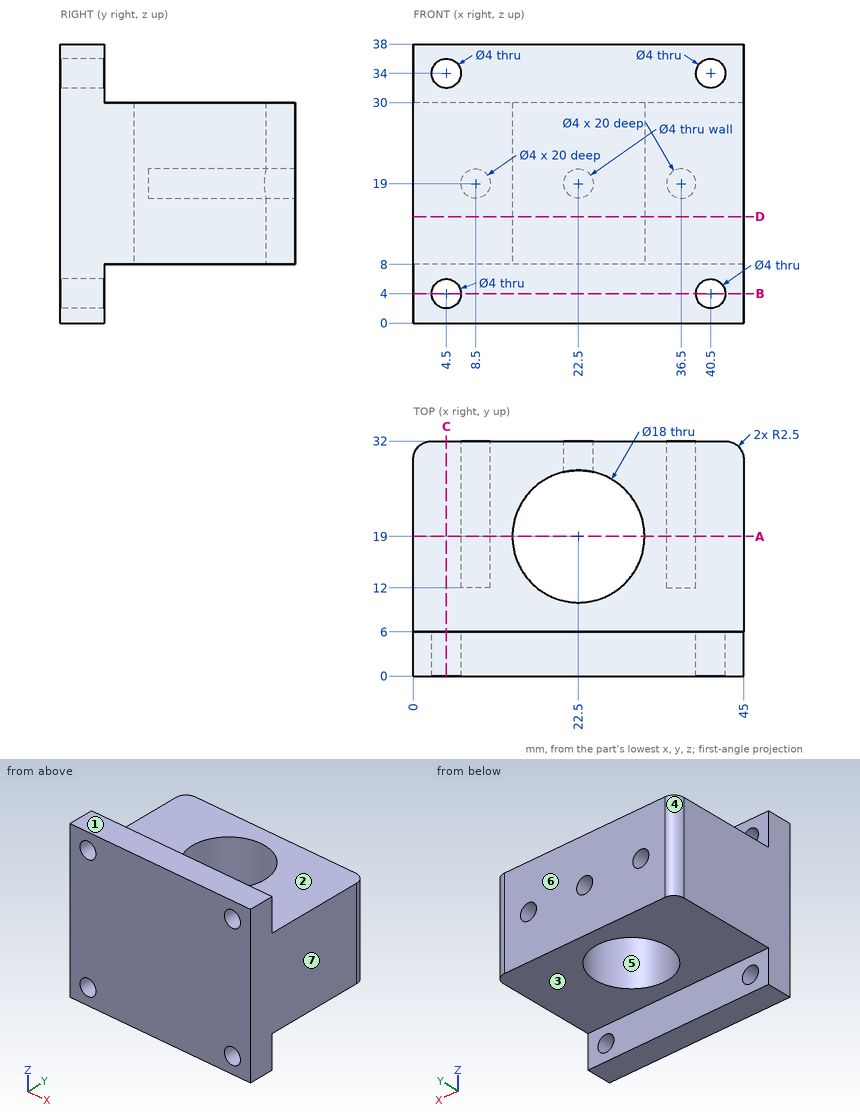
For this review, use the dimensioned drawing (mm, ordinates from the lowest corner) and the shaded views. A direction names the side the tool comes from. Coordinates: 2 decimals unless noted, no trailing zeros. Loops run counter-clockwise (first coordinate to the right, second up) from the corner with the lowest first, then second, coordinate; pieces in that order, holes last. Notation, with made-up numbers: (13, 29.5) - (49, 29.5) arc R30 cw to (49, 56.5) - close; hole circle Ø9 at (17, -16). An arc over 180 degrees is marked (long way). Use CSV: the item, a comma, the result in double quotes. Start each with the question number.
1) The part is to be moulded in two halves that separate along X. For the marked faces 4, 5, 6 and 7, say which applies: +X half, -X half, draft (parallel to the pull), parting line (faces both ways), or undercut.
2) Tool access review of the marked faces 1, 2 and 3: name each direction out of +Z, -Z, +X, -X, +Y, -Y from which nothing blocks a thin tool from reaching the whole face with its end or side.
3) Consider section A-A on y = 19. Write out the cut boundary in (x, z), then the cut area to 3 significant figures.
4) For pin 1 Ø5 at (x, z) = (40.5, 4) entering from -Y; pin 2 Ø1 at (x, y) = (32, 23) entering from -Z; pin 3 Ø9 at (x, z) = (11.5, 35.5) entering from +Y; pin 4 Ø1.2 at (x, z) = (9, 18) entering from +Y, all flat-tipped, find the tip position at first contact; note any pin that passes through.
5) Consider section B-B on z = 4. Write out the cut boundary in (x, y).
6) Wall thickness on L1, parallel to X at y = 2, z = 34; L2, parallel to X at y = 25.5, z = 19; L3, parallel to X at y = 29.35, z = 19: over which ranges is each line inside the solid? List them lowest first. Write a range as from..to.
7) Consider section C-C on x = 4.5. Write out the cut boundary in (y, z), then the cut area to 3 significant figures.
8) Consider section D-D on z = 14.5. Write out the cut boundary in (x, y).
Geometry says:
1,face 4,"-X half"
1,face 5,"undercut"
1,face 6,"draft"
1,face 7,"+X half"
2,face 1,"+Z, +X, -X, +Y, -Y"
2,face 2,"+Z, +X, -X, +Y"
2,face 3,"-Z, +X, -X, +Y"
3,outline,"(0, 8) - (13.5, 8) - (13.5, 30) - (0, 30) - close; (31.5, 8) - (45, 8) - (45, 30) - (31.5, 30) - close; hole circle Ø4 at (8.5, 19); hole circle Ø4 at (36.5, 19)"
3,area,"569 mm^2"
4,pin 1,"y = 0"
4,pin 2,"z = 8"
4,pin 3,"y = 6"
4,pin 4,"y = 12"
5,outline,"(0, 0) - (2.5, 0) - (2.5, 6) - (0, 6) - close; (6.5, 0) - (38.5, 0) - (38.5, 6) - (6.5, 6) - close; (42.5, 0) - (45, 0) - (45, 6) - (42.5, 6) - close"
6,L1,"0..2.5, 6.5..38.5, 42.5..45"
6,L2,"0..6.5, 10.5..16.28, 28.72..34.5, 38.5..45"
6,L3,"0..6.5, 10.5..20.5, 24.5..34.5, 38.5..45"
7,outline,"(0, 0) - (6, 0) - (6, 2) - (0, 2) - close; (0, 6) - (6, 6) - (6, 8) - (32, 8) - (32, 30) - (6, 30) - (6, 32) - (0, 32) - close; (0, 36) - (6, 36) - (6, 38) - (0, 38) - close"
7,area,"752 mm^2"
8,outline,"(0, 0) - (45, 0) - (45, 29.5) arc R2.5 ccw to (42.5, 32) - (2.5, 32) arc R2.5 ccw to (0, 29.5) - close; hole circle Ø18 at (22.5, 19)"
